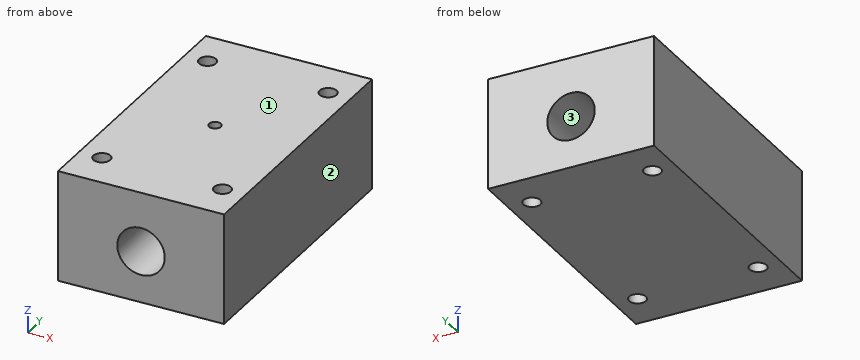
```python
from build123d import *

# Parameters (mm, degrees)
F0_W     = 42
F0_H     = 70
F0_R     = 2.15
F1_DEPTH = 28
F2_R     = 6
F3_DEPTH = 70
F4_R     = 1.5
F5_DEPTH = 5


with BuildPart() as f1:
    # F0 (on Top) → F1 (new body)
    with BuildSketch(Plane.XY):
        Rectangle(F0_W, F0_H)
        with Locations((-15.25, -25)):
            Circle(F0_R, mode=Mode.SUBTRACT)
        with Locations((15.25, -25)):
            Circle(F0_R, mode=Mode.SUBTRACT)
        with Locations((-15.25, 25)):
            Circle(F0_R, mode=Mode.SUBTRACT)
        with Locations((15.25, 25)):
            Circle(F0_R, mode=Mode.SUBTRACT)
    extrude(amount=-F1_DEPTH)

    # F2 (on face) → F3 (cut)
    with BuildSketch(Plane.XZ.offset(35)):
        with Locations((0, -15)):
            Circle(F2_R)
    extrude(amount=-F3_DEPTH, mode=Mode.SUBTRACT)

    # F4 (on face) → F5 (cut)
    with BuildSketch(Plane.XY):
        Circle(F4_R)
    extrude(amount=-F5_DEPTH, mode=Mode.SUBTRACT)


solid = f1.part
```
Build history of the part. All positions in model axes, mm. Face numbers are marked on the shaded views. Round coordinates to 2 decimals unless told otherwise and drop trailing zeros. Loops run counter-clockwise (first coordinate to the right, second up) from the corner with the lowest first, then second, coordinate; pieces in that order, holes last.
Item 1: Saw through at C-C (x = 0). List the corners of the cut face in (y, z), then the cut area to 4 significant figures.
Item 2: Saw through at B-B (z = -15). List the corners of the cut face in (x, y).
Item 3: Two-plate mould, pull along X, no slides. Class the marked faces 1, 2 and 3: released by +X, released by -X, zero draft, split by the parting line, or undercut.
Item 4: Drill centre lines: line 1 along Y through (x, z) = (-15.25, -17.75); line 2 along X through (y, z) = (26.5, -25.5); line 3 along Y through (x, z) = (14, -9). Where is each one in solid material? Low to high.
Item 5: Pin check, flat tip, straight feed: P1, Ø0.9, axis at x = 0, y = 0, coming from the +Z side. Stop position of the tip, or through.
Item 6: Saw through at D-D (y = 0). List the corners of the cut face in (x, z), then the cut area to 3 significant figures.
Item 7: Saw through at A-A (y = 25). List the corners of the cut face in (x, z), then the cut area to 3 significant figures.
Worked answers:
1. outline: (-35, -28) - (35, -28) - (35, -21) - (-35, -21) - close; (-35, -9) - (35, -9) - (35, 0) - (1.5, 0) - (1.5, -5) - (-1.5, -5) - (-1.5, 0) - (-35, 0) - close
1. area: 1,105 mm2
2. outline: (-21, -35) - (-6, -35) - (-6, 35) - (-21, 35) - close; (6, -35) - (21, -35) - (21, 35) - (6, 35) - close; hole circle Ø4.3 at (-15.25, -25); hole circle Ø4.3 at (-15.25, 25); hole circle Ø4.3 at (15.25, -25); hole circle Ø4.3 at (15.25, 25)
3. face 1: zero draft
3. face 2: released by +X
3. face 3: undercut
4. line 1: y = -35 to -27.15, -22.85 to 22.85, 27.15 to 35
4. line 2: x = -21 to -16.79, -13.71 to 13.71, 16.79 to 21
4. line 3: y = -35 to -26.75, -23.25 to 23.25, 26.75 to 35
5. P1: stops at z = -5
6. outline: (-21, -28) - (21, -28) - (21, 0) - (1.5, 0) - (1.5, -5) - (-1.5, -5) - (-1.5, 0) - (-21, 0) - close; hole circle Ø12 at (0, -15)
6. area: 1,050 mm2
7. outline: (-21, -28) - (-17.4, -28) - (-17.4, 0) - (-21, 0) - close; (-13.1, -28) - (13.1, -28) - (13.1, 0) - (-13.1, 0) - close; (17.4, -28) - (21, -28) - (21, 0) - (17.4, 0) - close; hole circle Ø12 at (0, -15)
7. area: 822 mm2
